Design review of the part built by this model. Coordinates are the model's own, in mm. A direction names the side the tool comes from. Round coordinates to 2 decimals unless told otherwise and drop trailing zeros. Order: outer loops, then holes, each group sorted by start corner. A loop starts at its lowest first (then second) coordinate and runs counter-clockwise, first axis right, second up. Notation, with made-up numbers: (12.25, 84) - (22.25, 84) arc R29 ccw to (22.25, 112) - close; hole circle Ø4 at (60.25, 67). An arc over 180 degrees is marked (long way). Write item = value, one per line.
from build123d import *

# Parameters (mm, degrees)
SKETCH_1_R          = 70
EXTRUDE_1_DEPTH     = 125
SKETCH_4_R          = 60
CUT_EXTRUDE_4_DEPTH = 110
SKETCH_5_R          = 61
CUT_EXTRUDE_5_DEPTH = 10
SKETCH_6_R          = 12.5
SKETCH_6_R_2        = 3
CUT_EXTRUDE_6_DEPTH = 152.739909055
SKETCH_7_R          = 60
SKETCH_7_R_2        = 50
EXTRUDE_2_DEPTH     = 5
SKETCH_8_R          = 2.5
CUT_EXTRUDE_7_DEPTH = 5


with BuildPart() as part:
    # 스케치1 → 보스-돌출1 (new body)
    with BuildSketch(Plane(origin=(0, 0, 0), x_dir=(1, 0, 0), z_dir=(0, 1, 0))):
        with Locations(Location((0, 0, 0), (0, 0, 270))):
            Circle(SKETCH_1_R)
    extrude(amount=EXTRUDE_1_DEPTH)

    # 스케치4 → 컷-돌출4 (cut)
    with BuildSketch(Plane.XZ):
        with Locations(Location((0, 0, 0), (0, 0, 270))):
            Circle(SKETCH_4_R)
    extrude(amount=-CUT_EXTRUDE_4_DEPTH, mode=Mode.SUBTRACT)

    # 스케치5 → 컷-돌출5 (cut)
    with BuildSketch(Plane(origin=(0, 125, 0), x_dir=(1, 0, 0), z_dir=(0, 1, 0))):
        with Locations(Location((0, 0, 0), (0, 0, 270))):
            Circle(SKETCH_5_R)
    extrude(amount=-CUT_EXTRUDE_5_DEPTH, mode=Mode.SUBTRACT)

    # 스케치6 → 컷-돌출6 (cut, through all)
    with BuildSketch(Plane(origin=(0, 115, 0), x_dir=(1, 0, 0), z_dir=(0, 1, 0))):
        with Locations(Location((0, 0, 0), (0, 0, 270))):
            Circle(SKETCH_6_R)
        with Locations(Location((0, -17.5, 0), (0, 0, 270))):
            Circle(SKETCH_6_R_2)
        with Locations(Location((-17.5, 0, 0), (0, 0, 270))):
            Circle(SKETCH_6_R_2)
        with Locations(Location((0, 17.5, 0), (0, 0, 270))):
            Circle(SKETCH_6_R_2)
        with Locations(Location((17.5, 0, 0), (0, 0, 270))):
            Circle(SKETCH_6_R_2)
    extrude(amount=-CUT_EXTRUDE_6_DEPTH, mode=Mode.SUBTRACT)

    # 스케치7 → 보스-돌출2 (add)
    with BuildSketch(Plane.XZ):
        with Locations(Location((0, 0, 0), (0, 0, 270))):
            Circle(SKETCH_7_R)
        with Locations(Location((0, 0, 0), (0, 0, 270))):
            Circle(SKETCH_7_R_2, mode=Mode.SUBTRACT)
    extrude(amount=-EXTRUDE_2_DEPTH)

    # 스케치8 → 컷-돌출7 (cut)
    with BuildSketch(Plane.XZ):
        with Locations(Location((0, -55, 0), (0, 0, 270))):
            Circle(SKETCH_8_R)
        with Locations(Location((-55, 0, 0), (0, 0, 270))):
            Circle(SKETCH_8_R)
        with Locations(Location((0, 55, 0), (0, 0, 270))):
            Circle(SKETCH_8_R)
        with Locations(Location((55, 0, 0), (0, 0, 270))):
            Circle(SKETCH_8_R)
    extrude(amount=-CUT_EXTRUDE_7_DEPTH, mode=Mode.SUBTRACT)


solid = part.part
1) Clearance check with flat-ended pins moving along their axes: pin 1 Ø7 at (x, z) = (0, 17.5) entering from +Y; pin 2 Ø4 at (y, z) = (66.5, -27) entering from -X; pin 3 Ø1.5 at (x, y) = (-26.5, 35) entering from +Z. State where each tip first meets the part, or that it passes through.
Findings:
pin_1 = 115
pin_2 = -65.38
pin_3 = 65.09
2) To check wall thickness, follow L1, parallel to X at y = 3.55, z = 0; L2, parallel to X at y = 121, z = 0; L3, parallel to X at y = 75, z = 0. State the ranges of each line that lie inside material, in increasing order. Write a range as from..to.
Findings:
L1 = -70..-57.5, -52.5..-50, 50..52.5, 57.5..70
L2 = -70..-61, 61..70
L3 = -70..-60, 60..70
3) We need section D-D on z = -55. Write out the cut boundary in (x, y), and give its area (3 significant figures).
Findings:
outline = (-43.3, 0) - (-2.5, 0) - (-2.5, 5) - (-23.98, 5) - (-23.98, 110) - (23.98, 110) - (23.98, 5) - (2.5, 5) - (2.5, 0) - (43.3, 0) - (43.3, 125) - (26.38, 125) - (26.38, 115) - (-26.38, 115) - (-26.38, 125) - (-43.3, 125) - close
area = 5,240 mm^2
4) We need section C-C on y = 36. Write out the cut boundary in (x, z).
Findings:
outline = circle Ø140 at (0, 0); hole circle Ø120 at (0, 0)
5) We need section B-B on x = 55. Write out the cut boundary in (y, z).
Findings:
outline = (0, -43.3) - (125, -43.3) - (125, -26.38) - (115, -26.38) - (115, 26.38) - (125, 26.38) - (125, 43.3) - (0, 43.3) - (0, 2.5) - (5, 2.5) - (5, 23.98) - (110, 23.98) - (110, -23.98) - (5, -23.98) - (5, -2.5) - (0, -2.5) - close
6) The part is to be moulded in two halves that separate along X. For faces 1 (the cylindrical face through (-42.594, 61.625, -55.55)), 2 (the flat face through (17, 0, 48)), 3 (the cylindrical face through (-20.43, 112.54, -0.65)), say which applies: released by +X, released by -X, zero draft, split by the parting line, or undercut.
Findings:
face_1 = split by the parting line
face_2 = zero draft
face_3 = undercut
7) For faces 4 (the cylindrical face through (-0.96, 2.46, -57.31)), 5 (the flat face through (14, 110, 1)), 6 (the cylindrical face through (3.755, 112.535, 11.923)), 7 (the flat face through (-13, 115, -1)), list the 3-axis set-ups (+Z, -Z, +X, -X, +Y, -Y) from which the entire face can be reached by the end or side of a thin tool; tool diameter is ignored.
Findings:
face_4 = -Y
face_5 = none
face_6 = +Y, -Y
face_7 = +Y
8) We need section A-A on z = -17.5. Write out the cut boundary in (x, y).
Findings:
outline = (-67.78, 0) - (-46.84, 0) - (-46.84, 5) - (-57.39, 5) - (-57.39, 110) - (-3, 110) - (-3, 115) - (-58.44, 115) - (-58.44, 125) - (-67.78, 125) - close; (3, 110) - (57.39, 110) - (57.39, 5) - (46.84, 5) - (46.84, 0) - (67.78, 0) - (67.78, 125) - (58.44, 125) - (58.44, 115) - (3, 115) - close
